```python
from build123d import *

# Parameters (mm, degrees)
SKETCH2_R           = 35
BOSS_EXTRUDE1_DEPTH = 5
SKETCH4_R           = 1.65
SKETCH4_W           = 60
SKETCH4_H           = 20
CUT_EXTRUDE1_DEPTH  = 5


with BuildPart() as part:
    # Sketch2 → Boss-Extrude1 (new body)
    with BuildSketch(Plane.XY):
        Circle(SKETCH2_R)
    extrude(amount=BOSS_EXTRUDE1_DEPTH)

    # Sketch4 → Cut-Extrude1 (cut)
    with BuildSketch(Plane.XY.offset(5)):
        with Locations((5, 3.9)):
            Circle(SKETCH4_R)
        with Locations((25, 3.9)):
            Circle(SKETCH4_R)
        with Locations((30, 25)):
            Rectangle(SKETCH4_W, SKETCH4_H)
    extrude(amount=-CUT_EXTRUDE1_DEPTH, mode=Mode.SUBTRACT)


solid = part.part
```
The listing builds one solid part. Answer for the finished solid, in the listing's coordinates (mm). A direction names the side the tool comes from. Give positions to 0.01 mm unless a question says otherwise; leave off trailing zeros. Order: outer loops, then holes, each group sorted by start corner. A loop starts at its lowest first (then second) coordinate and runs counter-clockwise, first axis right, second up. Notation, with made-up numbers: (1, 83.5) -> (52, 83.5) arc R30 cw to (52, 117.5) -> close; hole circle Ø10 at (11, 55.5). An arc over 180 degrees is marked (long way). Answer as a JSON object with one key per item and string values. Group by question number.
Item 1: A tool of negligible diameter and unlimited length cuts with its end or side. For faces 1 (the flat face through (0, 25, 3)), 2 (the flat face through (0, -7, 5)), from which of +Z, -Z, +X, -X, +Y, -Y can it reach the whole face along a straight path? Write none if from no direction.
Item 2: Consider L1, parallel to X at y = 5, z = 4.1; L2, parallel to Y at x = 6.5, z = 2; L3, parallel to Y at x = 25, z = 1.15. Determine where each line is inside the solid, lowest interval first. Write a range as from..to.
Item 3: The part is cut by section A-A on x = 5. Write down the section's boundary in (y, z).
Item 4: The part is cut by section C-C on y = 3.9. Write down the section's boundary in (x, z).
Item 5: Determine the mould class of faces 3 (the cylindrical face through (3.35, 3.97, 2.54)), 4 (the flat face through (0, -7, 0)), 5 (the cylindrical face through (-19.76, -28.89, 2.46)) for opening direction X: pulls with the +X half, pulls with the -X half, needs draft (parallel to the pull), parting line crosses it, or undercut.
Item 6: Flat-ended cylindrical pins translate along their axes: pin 1 (3 mm diameter, centred on y = 10, z = 1.5, fed in from -X); pin 2 (1.5 mm diameter, centred on x = 21, z = 3.5, fed in from +Y); pin 3 (2 mm diameter, centred on x = -2.5, z = 3, fed in from +Y). Find the tip coordinate at first contact, or state that the pin passes through.
Item 7: The part is cut by section D-D on x = 25. Write down the section's boundary in (y, z).
Item 8: The part is cut by section B-B on z = 3.4. Write down the section's boundary in (x, y).
Result set:
{
 "1": {"face 1": "+Z, -Z, +X, +Y", "face 2": "+Z, +X, -X, +Y, -Y"},
 "2": {"L1": "-34.64..3.77, 6.23..23.77, 26.23..34.64", "L2": "-34.39..3.21, 4.59..15", "L3": "-24.49..2.25, 5.55..15"},
 "3": {"outline": "(-34.64, 0) -> (2.25, 0) -> (2.25, 5) -> (-34.64, 5) -> close; (5.55, 0) -> (15, 0) -> (15, 5) -> (5.55, 5) -> close"},
 "4": {"outline": "(-34.78, 0) -> (3.35, 0) -> (3.35, 5) -> (-34.78, 5) -> close; (6.65, 0) -> (23.35, 0) -> (23.35, 5) -> (6.65, 5) -> close; (26.65, 0) -> (34.78, 0) -> (34.78, 5) -> (26.65, 5) -> close"},
 "5": {"face 3": "undercut", "face 4": "needs draft", "face 5": "parting line crosses it"},
 "6": {"pin 1": "x = -33.95", "pin 2": "y = 15", "pin 3": "y = 34.97"},
 "7": {"outline": "(-24.49, 0) -> (2.25, 0) -> (2.25, 5) -> (-24.49, 5) -> close; (5.55, 0) -> (15, 0) -> (15, 5) -> (5.55, 5) -> close"},
 "8": {"outline": "(0, 15) -> (0, 35) arc R35 ccw (long way) to (31.62, 15) -> close; hole circle Ø3.3 at (5, 3.9); hole circle Ø3.3 at (25, 3.9)"}
}
